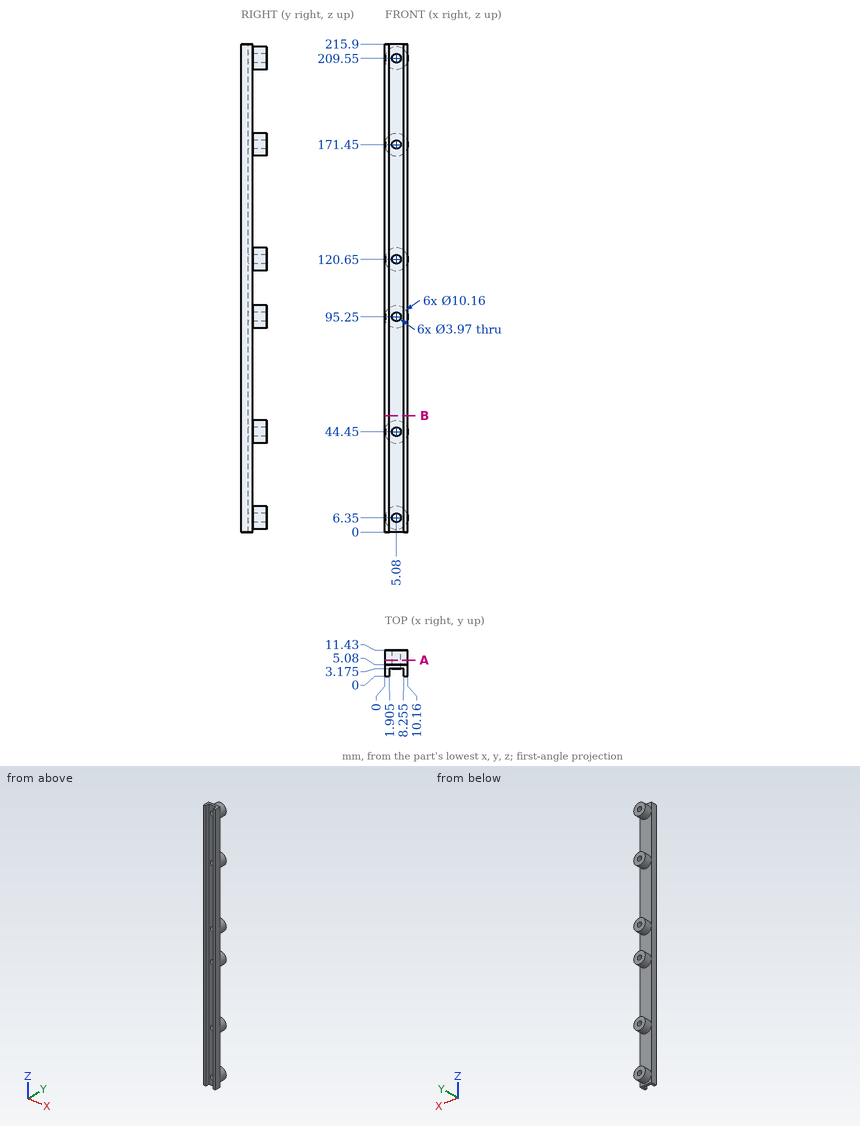
Geometry check sheet. Reference: drawing and pictorial views, mm from the part's lowest x, y, z. Coordinates: 2 decimals unless noted, no trailing zeros. Order: outer loops, then holes, each group sorted by start corner. A loop starts at its lowest first (then second) coordinate and runs counter-clockwise, first axis right, second up. Notation, with made-up numbers: (-6, 77.25) - (16, 77.25) arc R10 ccw to (16, 90.25) - close; hole circle Ø9 at (-11, -33.75). An arc over 180 degrees is marked (long way). One line per item, written item: value.
(1) Depth check by flat-ended pin: pin 1 Ø3 at (x, z) = (5.08, 6.35) entering from +Y; pin 2 Ø3 at (x, z) = (4.5, 190) entering from +Y; pin 3 Ø5 at (x, z) = (4.5, 144.5) entering from -Y (3 decimals). Enter the tip coordinate at first touch or a pass-through.
Data:
pin 1: passes through
pin 2: stops at y = 5.08
pin 3: stops at y = 3.175
(2) Sectioned sample at B-B (z = 51.5). Enter the section's corners in (x, y) (3 decimals).
Data:
outline: (0, 0) - (1.905, 0) - (1.905, 3.175) - (8.255, 3.175) - (8.255, 0) - (10.16, 0) - (10.16, 5.08) - (0, 5.08) - close
(3) Sectioned sample at A-A (y = 7). Count the separate pieces of the cut face and the enclosed holes in it, and give its area (3 significant figures).
Data:
separate pieces: 6
enclosed holes: 6
area: 412 mm^2
(4) Thickness scan on probe 1 along X at (y, z) = (5, 209.55) (3 decimals); probe 2 along X at (y, z) = (3, 177) (3 decimals); probe 3 along Z at (x, y) = (9.25, 8.75). Record the ranges inside material, lowest first. Write a range as from..to.
Data:
probe 1: x = 0..3.095, 7.065..10.16
probe 2: x = 0..1.905, 8.255..10.16
probe 3: z = 3.45..9.25, 41.55..47.35, 92.35..98.15, 117.75..123.55, 168.55..174.35, 206.65..212.45
